Model file for the job. Use its own axes, mm. A direction names the side the tool comes from. Give positions to 0.01 mm unless a question says otherwise; leave off trailing zeros. Write each loop counter-clockwise with the first axis right and the second up, starting at its lowest first coordinate (ties: lowest second). Pieces come first, ordered by that corner, then holes. Notation, with made-up numbers: (36.25, 0.25) - (64.25, 0.25) arc R16 cw to (64.25, 19.25) - close; hole circle Ø9 at (14.5, -36.5). An arc over 180 degrees is marked (long way). Use CSV: the item, a comma, the result in double quotes.
from build123d import *

# Parameters (mm, degrees)
CUT_EXTRUDE1_DEPTH      = 53.363441445
CUT_EXTRUDE1_DEPTH_BACK = 53.363441445


with BuildPart() as part:
    # Sketch1 → Revolve1 (revolve)
    with BuildSketch(Plane.XY, mode=Mode.PRIVATE) as revolve1_sk:
        with BuildLine():
            Line((12.7, 0), (12.7, 25.4))
            Line((12.7, 25.4), (16.51, 25.4))
            Line((16.51, 25.4), (16.51, 38.1))
            Line((16.51, 38.1), (21.59, 38.1))
            Line((21.59, 38.1), (21.59, 35.56))
            ThreePointArc((21.59, 35.56), (17.78, 31.75), (21.59, 27.94))
            Line((21.59, 27.94), (21.59, 25.4))
            Line((21.59, 25.4), (25.4, 25.4))
            Line((25.4, 25.4), (25.4, 0))
            Line((25.4, 0), (12.7, 0))
        make_face()
    revolve(revolve1_sk.sketch.rotate(Axis((0, 0, 0), (0, 1, 0)), 90), axis=Axis((0, 0, 0), (0, 1, 0)))

    # Sketch2 → Cut-Extrude1 (cut, two sides: drawn at the far end of the back side and taken through both)
    with BuildSketch(Plane(origin=(0, 0, 0), x_dir=(0, 0, -1), z_dir=(1, 0, 0)).offset(-CUT_EXTRUDE1_DEPTH_BACK)):
        Polygon((0, 20.32), (-6.599113577, 16.51), (-6.599113577, 8.89), (0, 5.08), (6.599113577, 8.89), (6.599113577, 16.51), align=None)
    extrude(amount=CUT_EXTRUDE1_DEPTH + CUT_EXTRUDE1_DEPTH_BACK, mode=Mode.SUBTRACT)


solid = part.part
(1) Pull direction X, two halves, no side cores. Call faces 1 (the face through (14.647, 31.839, -7.618)), 2 (the face through (18.024, 6.958, -3.253)), 3 (the face through (9.728, 12.522, -23.463)): released by +X, released by -X, zero draft, split by the parting line, or undercut.
Checked values:
face 1,"undercut"
face 2,"zero draft"
face 3,"split by the parting line"
(2) Flat gauge pins, fed straight in: P1, Ø8.5, axis at x = 19.5, y = 13, coming from the +Z side; P2, Ø16.5, axis at x = -6.5, z = -0.5, coming from the +Y side; P3, Ø6, axis at x = -16.5, y = 11, coming from the -Z side; P4, Ø3, axis at x = 12, z = -5, coming from the -Y side. Where does each tip first touch, or does it go through?
Checked values:
P1,"stops at z = 20.31"
P2,"stops at y = 25.4"
P3,"stops at z = -21.52"
P4,"stops at y = 0"
(3) Saw through at D-D, the plane z = 3. Count the separate pieces of the cut face and the enclosed holes in it, then the cut area to 3 significant figures.
Checked values:
separate pieces,"4"
enclosed holes,"0"
area,"436 mm^2"
(4) Wall check: probe 1 along Y at (x, z) = (-18.5, -2.5); probe 2 along Y at (x, z) = (5, -13); probe 3 along X at (y, z) = (31, -12.5). Give the ranges that are in metal, low to high. Write a range as [from, to].
Checked values:
probe 1,"y = [0, 6.52], [18.88, 29.3], [34.2, 38.1]"
probe 2,"y = [0, 25.4]"
probe 3,"x = [-12.75, -10.79], [10.79, 12.75]"
(5) Saw through at C-C, the plane y = 4. List the corners of the cut face in (x, z), then the cut area to 3 significant figures.
Checked values:
outline,"circle Ø50.8 at (0, 0); hole circle Ø25.4 at (0, 0)"
area,"1,520 mm^2"
(6) 3-axis set-ups, long thin cutter, end or side, ignore diameter. For faces 4 (the face through (-18, 13, 6.599)), 5 (the face through (-14.592, 26.652, 15.913)), 6 (the face through (16, 38.1, -5)): which of +Z, -Z, +X, -X, +Y, -Y reach the whole face in a straight line?
Checked values:
face 4,"+X, -X"
face 5,"+Y"
face 6,"+Z, -Z, +X, -X, +Y"
(7) Saw through at A-A, the plane y = 10.5. List the corners of the cut face in (x, z), then the cut area to 3 significant figures.
Checked values:
outline,"(-24.53, -6.6) arc R25.4 ccw to (24.53, -6.6) - (10.85, -6.6) arc R12.7 cw to (-10.85, -6.6) - close; (-24.53, 6.6) - (-10.85, 6.6) arc R12.7 cw to (10.85, 6.6) - (24.53, 6.6) arc R25.4 ccw to start"
area,"1,180 mm^2"
(8) Saw through at B-B, the plane x = 0. List the corners of the cut face in (y, z).
Checked values:
outline,"(0, -25.4) - (25.4, -25.4) - (25.4, -21.59) - (27.94, -21.59) arc R3.81 cw to (35.56, -21.59) - (38.1, -21.59) - (38.1, -16.51) - (25.4, -16.51) - (25.4, -12.7) - (0, -12.7) - close; (0, 12.7) - (25.4, 12.7) - (25.4, 16.51) - (38.1, 16.51) - (38.1, 21.59) - (35.56, 21.59) arc R3.81 cw to (27.94, 21.59) - (25.4, 21.59) - (25.4, 25.4) - (0, 25.4) - close"
